Here's how the part is built. I have some questions about the finished solid (model axes, mm). Face numbers are marked on the shaded views. A direction names the side the tool comes from. Give positions to 0.01 mm unless a question says otherwise; leave off trailing zeros. Write each loop counter-clockwise with the first axis right and the second up, starting at its lowest first coordinate (ties: lowest second). Pieces come first, ordered by that corner, then holes. Notation, with made-up numbers: (76, 59) -> (114, 59) arc R33 ccw to (114, 98) -> close; hole circle Ø7 at (-29.75, 55). An arc over 180 degrees is marked (long way). Return JSON: item names as keys, results as strings.
from build123d import *

# Parameters (mm, degrees)
SKETCH1_W           = 44.5
SKETCH1_H           = 30
BOSS_EXTRUDE1_DEPTH = 12.5
SHELL2_T            = 1.2
SKETCH2_W           = 5
SKETCH2_H           = 5.5
CUT_EXTRUDE1_DEPTH  = 1.2
SKETCH3_W           = 4.2
SKETCH3_H           = 5
CUT_EXTRUDE2_DEPTH  = 1.2
FILLET1_R           = 5
FILLET3_R           = 1


with BuildPart() as part:
    # Sketch1 → Boss-Extrude1 (new body)
    with BuildSketch(Plane(origin=(0, 0, 0), x_dir=(0, 0, -1), z_dir=(1, 0, 0))):
        Rectangle(SKETCH1_W, SKETCH1_H)
    extrude(amount=BOSS_EXTRUDE1_DEPTH)

    # Shell2
    shell2_openings = [part.faces().sort_by_distance(p)[0] for p in [
        (0, 0, 0),
    ]]
    offset(amount=SHELL2_T, openings=shell2_openings, kind=Kind.INTERSECTION)

    # Sketch2 → Cut-Extrude1 (cut)
    with BuildSketch(Plane.XZ.offset(-15)):
        with Locations((2.5, 17)):
            Rectangle(SKETCH2_W, SKETCH2_H)
        with Locations((2.5, 8.5)):
            Rectangle(SKETCH2_W, SKETCH2_H)
        with Locations((2.5, 0)):
            Rectangle(SKETCH2_W, SKETCH2_H)
        with Locations((2.5, -8.5)):
            Rectangle(SKETCH2_W, SKETCH2_H)
    extrude(amount=-CUT_EXTRUDE1_DEPTH, mode=Mode.SUBTRACT)

    # Sketch3 → Cut-Extrude2 (cut)
    with BuildSketch(Plane(origin=(0, 0, -23.45), x_dir=(-1, 0, 0), z_dir=(0, 0, -1))):
        with BuildLine():
            Line((0, 3), (-1.95, 3))
            ThreePointArc((-1.95, 3), (-4.2, 0.75), (-1.95, -1.5))
            Line((-1.95, -1.5), (0, -1.5))
            Line((0, -1.5), (0, 3))
        make_face()
        with Locations((-2.1, 9.5)):
            Rectangle(SKETCH3_W, SKETCH3_H)
    extrude(amount=-CUT_EXTRUDE2_DEPTH, mode=Mode.SUBTRACT)

    # Fillet1
    fillet1_edges = [part.edges().sort_by_distance(p)[0] for p in [
        (13.7, -16.2, 0),
        (12.5, 15, 0),
        (12.5, -15, 0),
        (13.7, 16.2, 0),
    ]]
    fillet(fillet1_edges, radius=FILLET1_R)

    # Fillet3
    fillet3_edges = [part.edges().sort_by_distance(p)[0] for p in [
        (13.7, 0, -23.45),
        (13.7, 0, 23.45),
        (4.35, 16.2, -23.45),
        (4.35, -16.2, -23.45),
        (12.235533906, 14.735533906, -23.45),
        (12.235533906, -14.735533906, -23.45),
        (4.35, -16.2, 23.45),
        (4.35, 16.2, 23.45),
        (12.235533906, 14.735533906, 23.45),
        (12.235533906, -14.735533906, 23.45),
    ]]
    fillet(fillet3_edges, radius=FILLET3_R)


solid = part.part
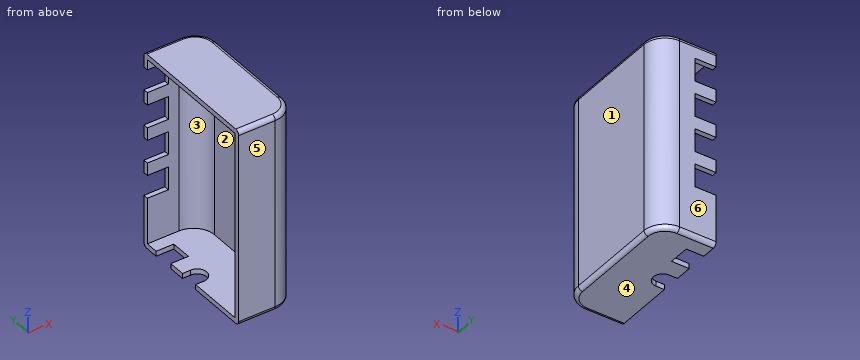
1. If I drill on line 1 (Y direction, x = 5.75, z = 11); line 2 (Z direction, x = 11.5, y = -6); line 3 (X direction, y = 1.5, z = -13), over which ranges is the centre line in solid material (lowest first)? Write a range as [from, to].
Taken from the geometry:
{"line 1": "y = [-16.2, -15], [15, 16.2]", "line 2": "z = [-23.45, -22.25], [22.25, 23.45]", "line 3": "x = [12.5, 13.7]"}
2. Suppose I cut it at D-D, the plane x = 1.25. Count the separate pieces of the cut face and the enclosed holes in it, and give its area (3 significant figures).
Taken from the geometry:
{"separate pieces": "6", "enclosed holes": "0", "area": "146 mm²"}
3. Suppose I cut it at B-B, the plane z = 9.5. List the corners of the cut face in (x, y) for me.
Taken from the geometry:
{"outline": "(0, -16.2) -> (8.7, -16.2) arc R5 ccw to (13.7, -11.2) -> (13.7, 11.2) arc R5 ccw to (8.7, 16.2) -> (5, 16.2) -> (5, 15) -> (7.5, 15) arc R5 cw to (12.5, 10) -> (12.5, -10) arc R5 cw to (7.5, -15) -> (0, -15) -> close"}
4. Suppose I cut it at C-C, the plane y = 0.75. List the corners of the cut face in (x, z) for me, and give its area (3 significant figures).
Taken from the geometry:
{"outline": "(0, 22.25) -> (12.5, 22.25) -> (12.5, -22.25) -> (4.2, -22.25) -> (4.2, -23.45) -> (12.7, -23.45) arc R1 ccw to (13.7, -22.45) -> (13.7, 22.45) arc R1 ccw to (12.7, 23.45) -> (0, 23.45) -> close", "area": "80.8 mm²"}
5. Suppose I cut it at A-A, the plane x = 7. List the corners of the cut face in (y, z) for me.
Taken from the geometry:
{"outline": "(-16.2, -22.45) arc R1 ccw to (-15.2, -23.45) -> (15.2, -23.45) arc R1 ccw to (16.2, -22.45) -> (16.2, 22.45) arc R1 ccw to (15.2, 23.45) -> (-15.2, 23.45) arc R1 ccw to (-16.2, 22.45) -> close; hole (-15, -22.25) -> (15, -22.25) -> (15, 22.25) -> (-15, 22.25) -> close"}
6. Which directions (+Z, -Z, +X, -X, +Y, -Y) give clear straight access to the entire face, cutting with the end or side of a thin tool? Please do the marked faces 1 and 2.
Taken from the geometry:
{"face 1": "+Z, -Z, +X, +Y, -Y", "face 2": "-X"}
7. If we mould it in two halves opening along Y, with no side actions, what happens to the marked faces 3, 4, 5 and 6? For each: released by +Y, released by -Y, zero draft, split by the parting line, or undercut.
Taken from the geometry:
{"face 3": "undercut", "face 4": "zero draft", "face 5": "released by -Y", "face 6": "released by +Y"}
8. For pin 1 Ø1 at (x, z) = (1.5, -23) entering from -Y; pin 2 Ø16 at (y, z) = (2.5, -4) entering from -X; pin 3 Ø4 at (y, z) = (10, -16.5) entering from -X; pin 4 Ø0.6 at (x, z) = (0.5, -23) entering from +Y, each with a flat end and sliding along its axis, tell me the tip position at first contact or that it passes through.
Taken from the geometry:
{"pin 1": "stops at y = -16.2", "pin 2": "stops at x = 12.47", "pin 3": "stops at x = 12.08", "pin 4": "stops at y = 16.17"}
